```python
from build123d import *

# Parameters (mm, degrees)
F0_W     = 76.2
F0_H     = 25.4
F1_DEPTH = 38.1
F2_W     = 66.802
F2_H     = 13.208
F3_DEPTH = 16.002
F4_R     = 6.35
F5_R     = 4.7752
F6_R     = 4.7752
F8_D     = 4.0386
F8_DEPTH = 12.7
F8_TIP   = 1.213317848


with BuildPart() as f1:
    # F0 (on Top) → F1 (new body)
    with BuildSketch(Plane.XY):
        Rectangle(F0_W, F0_H)
    extrude(amount=F1_DEPTH)

    # F2 (on face) → F3 (cut)
    with BuildSketch(Plane.XZ.offset(12.7)):
        with Locations((-4.699, 31.496)):
            Rectangle(F2_W, F2_H)
        with Locations((-4.699, 6.604)):
            Rectangle(F2_W, F2_H)
    extrude(amount=-F3_DEPTH, mode=Mode.SUBTRACT)

    # F4
    f4_edges = [f1.edges().sort_by_distance(p)[0] for p in [
        (28.702, 3.302, 6.604),
        (28.702, 3.302, 31.496),
    ]]
    fillet(f4_edges, radius=F4_R)

    # F5
    f5_edges = [f1.edges().sort_by_distance(p)[0] for p in [
        (33.401, -12.7, 38.1),
        (33.401, -12.7, 0),
    ]]
    fillet(f5_edges, radius=F5_R)

    # F6
    f6_edges = [f1.edges().sort_by_distance(p)[0] for p in [
        (-38.1, -12.7, 19.05),
        (-38.1, 8.001, 38.1),
        (-38.1, 8.001, 0),
    ]]
    fillet(f6_edges, radius=F6_R)

    # F8
    with Locations(Plane.YZ.offset(38.1)):
        with Locations((-8.001, 4.826), (-8.001, 33.401), (7.874, 33.401), (7.874, 4.826)):
            Hole(F8_D / 2, depth=F8_DEPTH)
            with Locations((0, 0, -(F8_DEPTH + F8_TIP / 2))):  # 118° drill point
                Cone(0, F8_D / 2, F8_TIP, mode=Mode.SUBTRACT)


solid = f1.part
```
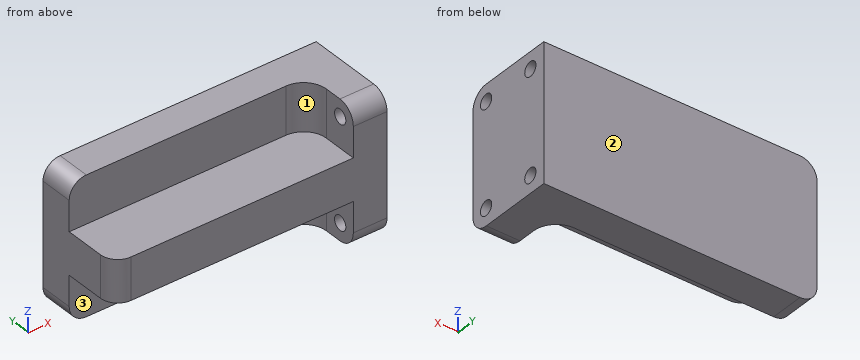
CAD build for the part. Positions are in the model's coordinates, mm. Face numbers are marked on the shaded views. A direction names the side the tool comes from. Round coordinates to 2 decimals unless told otherwise and drop trailing zeros. Write each loop counter-clockwise with the first axis right and the second up, starting at its lowest first coordinate (ties: lowest second). Pieces come first, ordered by that corner, then holes. Notation, with made-up numbers: (86, 4) -> (101, 4) arc R36 cw to (101, 39) -> close; hole circle Ø9 at (86.25, -11). An arc over 180 degrees is marked (long way). Answer in a Markdown table with one row per item. Add a question column.
Item 1: Drop flat-ended pins along their axis: pin 1 Ø8 at (x, y) = (-4.5, -5) entering from -Z; pin 2 Ø6.5 at (y, z) = (-8.001, 33.401) entering from -X; pin 3 Ø3.5 at (y, z) = (7.874, 4.826) entering from +X. Give the stop position or say it passes through.
Item 2: Saw through at B-B, the plane y = -4.25. Write the cut outline in (x, z), then the cut area to 3 significant figures.
Item 3: Drill centre lines: line 1 (Z direction, x = 32, y = 7); line 2 (Y direction, x = 29, z = 4); line 3 (Y direction, x = 5.5, z = 36.5). Where is each one in solid material? Low to high. Write a range as from..to.
Item 4: Which spindle directions (+Z, -Z, +X, -X, +Y, -Y) get a long thin tool onto all of the face, cutting with end or side? Do the marked faces 1, 2 and 3. Say none if no direction does.
Item 5: Saw through at C-C, the plane z = 29. Write the cut outline in (x, y), then the cut area to 3 significant figures.
Item 6: Saw through at A-A, the plane x = -21. Write the cut outline in (y, z), then the cut area to 3 significant figures.
Findings below:
| question | item | result |
|---|---|---|
| 1 | pin 1 | stops at z = 13.21 |
| 1 | pin 2 | stops at x = 28.7 |
| 1 | pin 3 | stops at x = 25.24 |
| 2 | outline | (-38.1, 13.21) -> (28.7, 13.21) -> (28.7, 0) -> (38.1, 0) -> (38.1, 38.1) -> (28.7, 38.1) -> (28.7, 24.89) -> (-38.1, 24.89) -> close |
| 2 | area | 1,140 mm^2 |
| 3 | line 1 | z = 0..3.01, 6.65..31.58, 35.22..38.1 |
| 3 | line 2 | y = -12.64..-9.84, -6.16..6.03, 9.72..12.7 |
| 3 | line 3 | y = 3.3..12.7 |
| 4 | face 1 | +Z, -X, -Y |
| 4 | face 2 | +Z, -Z, +X, -X, +Y |
| 4 | face 3 | -Z, -X, -Y |
| 5 | outline | (-38.1, 3.3) -> (22.35, 3.3) arc R6.35 cw to (28.7, -3.05) -> (28.7, -12.7) -> (38.1, -12.7) -> (38.1, 12.7) -> (-38.1, 12.7) -> close |
| 5 | area | 875 mm^2 |
| 6 | outline | (-12.7, 13.21) -> (3.3, 13.21) -> (3.3, 0) -> (12.7, 0) -> (12.7, 38.1) -> (3.3, 38.1) -> (3.3, 24.89) -> (-12.7, 24.89) -> close |
| 6 | area | 545 mm^2 |
